Here's how the part is built. I have some questions about the finished solid (model axes, mm). Face numbers are marked on the shaded views. A direction names the side the tool comes from. Round coordinates to 2 decimals unless told otherwise and drop trailing zeros. Loops run counter-clockwise (first coordinate to the right, second up) from the corner with the lowest first, then second, coordinate; pieces in that order, holes last. Notation, with made-up numbers: M 10.25,49.5 L 61.25,49.5 A12 ccw 61.25,59.5 Z; hole C 62.25,63.5 d8. An arc over 180 degrees is marked long. Answer as CSV lines item,"result".
```python
from build123d import *

# Parameters (mm, degrees)
TUBE_FULL_AF_EXTRUSION_DEPTH    = 201
TUBE_BORE_CUT_DEPTH             = 202.504085463
TUBE_BORE_CUT_DEPTH_BACK        = 202.504085463
T4_LOWER_BODY_RELIEF_START      = -6
T4_LOWER_BODY_RELIEF_DEPTH      = 9
T4_UPPER_BODY_RELIEF_START      = 6
T4_UPPER_BODY_RELIEF_DEPTH      = 180
T4_BOTTOM_END_CHAMFER_SIZE      = 0.8
T4_TUBE_MOUTH_CHAMFER_SIZE      = 0.8
T4_GUIDE_BAND_CORNER_FILLETS_R  = 0.5
T4_STOP_BAND_CORNER_FILLETS_R   = 0.5
T4_GUIDE_BAND_RIB_PROFILE_W     = 0.5
T4_GUIDE_BAND_RIB_PROFILE_H     = 5.2
T4_GUIDE_BAND_RIBS_MASTER_DEPTH = 0.15
T4_GUIDE_BAND_RIB_PATTERN_COUNT = 6


with BuildPart() as part:
    # Tube_Full_AF_Profile → Tube_Full_AF_Extrusion (new body)
    with BuildSketch(Plane.XY):
        Polygon((5.38379126, 9.325), (-5.38379126, 9.325), (-10.76758252, 0), (-5.38379126, -9.325), (5.38379126, -9.325), (10.76758252, 0), align=None)
    extrude(amount=TUBE_FULL_AF_EXTRUSION_DEPTH)

    # Tube_Bore_Profile → Tube_Bore_Cut (cut, two sides: drawn at the far end of the back side and taken through both)
    with BuildSketch(Plane.XY.offset(201).offset(-TUBE_BORE_CUT_DEPTH_BACK)):
        Polygon((8.458181444, 0), (4.229090722, 7.325), (-4.229090722, 7.325), (-8.458181444, 0), (-4.229090722, -7.325), (4.229090722, -7.325), align=None)
    extrude(amount=TUBE_BORE_CUT_DEPTH + TUBE_BORE_CUT_DEPTH_BACK, mode=Mode.SUBTRACT)

    # T4_Lower_Relief_Profile → T4_Lower_Body_Relief (cut)
    with BuildSketch(Plane.XY.offset(201).offset(T4_LOWER_BODY_RELIEF_START)):
        Polygon((10.76758252, 0), (5.38379126, 9.325), (-5.38379126, 9.325), (-10.76758252, 0), (-5.38379126, -9.325), (5.38379126, -9.325), align=None)
        Polygon((10.074762197, 0), (5.037381099, 8.725), (-5.037381099, 8.725), (-10.074762197, 0), (-5.037381099, -8.725), (5.037381099, -8.725), align=None, mode=Mode.SUBTRACT)
    extrude(amount=-T4_LOWER_BODY_RELIEF_DEPTH, mode=Mode.SUBTRACT)

    # T4_Upper_Relief_Profile → T4_Upper_Body_Relief (cut)
    with BuildSketch(Plane.XY.offset(174).offset(T4_UPPER_BODY_RELIEF_START)):
        Polygon((-5.38379126, -9.325), (5.38379126, -9.325), (10.76758252, 0), (5.38379126, 9.325), (-5.38379126, 9.325), (-10.76758252, 0), align=None)
        Polygon((5.037381099, -8.725), (10.074762197, 0), (5.037381099, 8.725), (-5.037381099, 8.725), (-10.074762197, 0), (-5.037381099, -8.725), align=None, mode=Mode.SUBTRACT)
    extrude(amount=-T4_UPPER_BODY_RELIEF_DEPTH, mode=Mode.SUBTRACT)

    # T4_Bottom_End_Chamfer
    t4_bottom_end_chamfer_edges = [part.edges().sort_by_distance(p)[0] for p in [
        (-8.07568689, 4.6625, 201),
        (-8.07568689, -4.6625, 201),
        (0, -9.325, 201),
        (8.07568689, -4.6625, 201),
        (8.07568689, 4.6625, 201),
        (0, 9.325, 201),
    ]]
    chamfer(t4_bottom_end_chamfer_edges, length=T4_BOTTOM_END_CHAMFER_SIZE)

    # T4_Tube_Mouth_Chamfer
    t4_tube_mouth_chamfer_edges = [part.edges().sort_by_distance(p)[0] for p in [
        (6.343636083, -3.6625, 0),
        (0, -7.325, 0),
        (-6.343636083, -3.6625, 0),
        (-6.343636083, 3.6625, 0),
        (0, 7.325, 0),
        (6.343636083, 3.6625, 0),
    ]]
    chamfer(t4_tube_mouth_chamfer_edges, length=T4_TUBE_MOUTH_CHAMFER_SIZE)

    # T4_Guide_Band_Corner_Fillets
    t4_guide_band_corner_fillets_edges = [part.edges().sort_by_distance(p)[0] for p in [
        (5.38379126, 9.325, 197.6),
        (-5.38379126, 9.325, 197.6),
        (-10.76758252, 0, 197.6),
        (-5.38379126, -9.325, 197.6),
        (5.38379126, -9.325, 197.6),
        (10.76758252, 0, 197.6),
    ]]
    fillet(t4_guide_band_corner_fillets_edges, radius=T4_GUIDE_BAND_CORNER_FILLETS_R)

    # T4_Stop_Band_Corner_Fillets
    t4_stop_band_corner_fillets_edges = [part.edges().sort_by_distance(p)[0] for p in [
        (10.76758252, 0, 183),
        (5.38379126, -9.325, 183),
        (-5.38379126, -9.325, 183),
        (-10.76758252, 0, 183),
        (-5.38379126, 9.325, 183),
        (5.38379126, 9.325, 183),
    ]]
    fillet(t4_stop_band_corner_fillets_edges, radius=T4_STOP_BAND_CORNER_FILLETS_R)

    # T4_Guide_Band_Rib_Profile → T4_Guide_Band_Ribs_Master (add)
    with BuildSketch(Plane(origin=(0, 9.325, 0), x_dir=(1, 0, 0), z_dir=(0, 1, 0))):
        with Locations((-4.75, -197.6)):
            Rectangle(T4_GUIDE_BAND_RIB_PROFILE_W, T4_GUIDE_BAND_RIB_PROFILE_H)
        with Locations((4.75, -197.6)):
            Rectangle(T4_GUIDE_BAND_RIB_PROFILE_W, T4_GUIDE_BAND_RIB_PROFILE_H)
    t4_guide_band_ribs_master = extrude(amount=T4_GUIDE_BAND_RIBS_MASTER_DEPTH)

    # T4_Guide_Band_Rib_Pattern: T4_Guide_Band_Ribs_Master ×6 about axis
    t4_guide_band_rib_pattern_axis = Axis((0, 0, 0), (0, 0, 1))
    for i in range(1, T4_GUIDE_BAND_RIB_PATTERN_COUNT):
        add(t4_guide_band_ribs_master.rotate(t4_guide_band_rib_pattern_axis, i * 360 / T4_GUIDE_BAND_RIB_PATTERN_COUNT))


solid = part.part
```
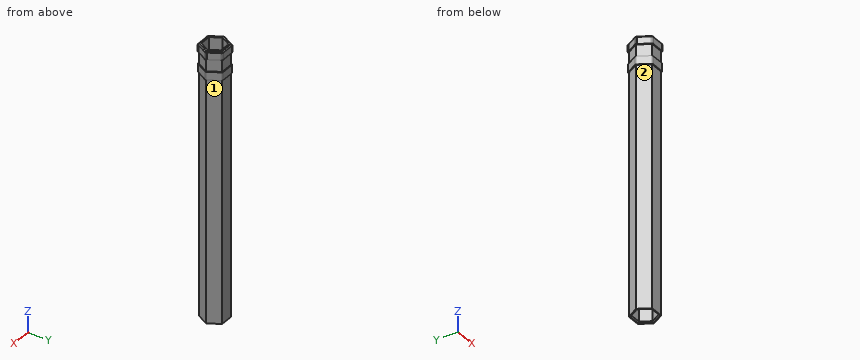
1. For P1, Ø9.5, axis at x = -5, y = -0.5, coming from the +Z side; P2, Ø8, axis at y = -4.5, z = 152, coming from the +X side; P3, Ø6, axis at x = -2, z = 157, coming from the -Y side (3 decimals); P4, Ø6.5, axis at x = 1, z = 182, coming from the -Y side (3 decimals), each with a flat end and sliding along its axis, tell me the tip position at first contact or that it passes through.
Evaluation:
P1,"stops at z = 201"
P2,"stops at x = 9.79"
P3,"stops at y = -8.725"
P4,"stops at y = -9.325"
2. I want a section at A-A, the plane x = 2.5. Please give me the cut outline in (y, z) (3 decimals).
Evaluation:
outline,"M -9.325,180 L -8.725,180 L -8.725,0 L -8.125,0 L -7.325,0.8 L -7.325,201 L -8.525,201 L -9.325,200.2 L -9.325,195 L -8.725,195 L -8.725,186 L -9.325,186 Z; M 7.325,0.8 L 8.125,0 L 8.725,0 L 8.725,180 L 9.325,180 L 9.325,186 L 8.725,186 L 8.725,195 L 9.325,195 L 9.325,200.2 L 8.525,201 L 7.325,201 Z"
3. Which directions (+Z, -Z, +X, -X, +Y, -Y) give clear straight access to the entire face, cutting with the end or side of a thin tool? Please do the marked faces 1 and 2.
Evaluation:
face 1,"-Z, +X, +Y"
face 2,"-Z, -X, -Y"
4. I want a section at B-B, the plane z = 47.5. Please give me the cut outline in (x, y) (3 decimals).
Evaluation:
outline,"M -10.075,0 L -5.037,-8.725 L 5.037,-8.725 L 10.075,0 L 5.037,8.725 L -5.037,8.725 Z; hole M -8.458,0 L -4.229,-7.325 L 4.229,-7.325 L 8.458,0 L 4.229,7.325 L -4.229,7.325 Z"
5. I want a section at C-C, the plane y = -2.75. Please give me the cut outline in (x, z).
Evaluation:
outline,"M -9.18,180 L -8.49,180 L -8.49,0 L -7.79,0 L -6.87,0.8 L -6.87,201 L -8.26,201 L -9.18,200.2 L -9.18,195 L -8.49,195 L -8.49,186 L -9.18,186 Z; M 6.87,0.8 L 7.79,0 L 8.49,0 L 8.49,180 L 9.18,180 L 9.18,186 L 8.49,186 L 8.49,195 L 9.18,195 L 9.18,200.2 L 8.26,201 L 6.87,201 Z"
6. If I drill on line 1 (Y direction, x = -1.5, z = 177) (3 decimals); line 2 (Y direction, x = -5, z = 101) (3 decimals); line 3 (X direction, y = -7.75, z = 47), over which ranges is the centre line in solid material (lowest first)? Write a range as [from, to].
Evaluation:
line 1,"y = [-8.725, -7.325], [7.325, 8.725]"
line 2,"y = [-8.725, -5.99], [5.99, 8.725]"
line 3,"x = [-5.6, 5.6]"
